Check sheet for the modelled part. Datum: model origin and axes. Units: mm. A direction names the side the tool comes from. Give positions to 0.01 mm unless a question says otherwise; leave off trailing zeros. Loops run counter-clockwise (first coordinate to the right, second up) from the corner with the lowest first, then second, coordinate; pieces in that order, holes last. Notation, with made-up numbers: (55, 28) -> (64, 28) arc R25 ccw to (64, 58) -> close; hole circle Ø8 at (40.25, 57). An arc over 180 degrees is marked (long way). Write each question's results on one line, items separated by ' | '. Start each with the question number.
Item 1: Cross-section at A-A on z = 0.5. Enter the section's corners in (x, y).
Item 2: Cross-section at B-B on y = 73. Enter the section's corners in (x, z).
Item 3: Mould release check, pull along Z, two halves, no side actions. Record for faces 3 (the face through (151.457, 44.37, 0.192)), 4 (the face through (121.87, 45.63, 12.22)), 5 (the face through (126.47, 44.37, 0.02)), 6 (the face through (-53.53, 44.37, 0.02)): pulls with the +Z half, pulls with the -Z half, needs draft (parallel to the pull), parting line crosses it, or undercut.
Item 4: Gauge pin test, flat ends, axial feed: pin 1 Ø1 at (x, y) = (84, 37.5) entering from +Z; pin 2 Ø4 at (y, z) = (52.5, -2.5) entering from -X; pin 3 Ø6 at (y, z) = (68.5, 11.5) entering from +X. Record the tip position at first contact, or that the pin passes through.
Item 5: Cross-section at D-D on z = 9.5. Enter the section's corners in (x, y).
Item 6: Cross-section at C-C on x = -36. Enter the section's corners in (y, z).
Item 7: Access from +Z, -Z, +X, -X, +Y, -Y to the whole of each face (thin tool, end or side, straight path). Record for faces 1 (the face through (48, 90, -12)), 2 (the face through (119.461, 44, -2)).
Item 8: Scan lines: line 1 along X through (y, z) = (25.5, 0.5); line 2 along X through (y, z) = (29, 8.5); line 3 along Z through (x, y) = (101, 52). Record each from-to range of solid material in increasing order.
from build123d import *

# Parameters (mm, degrees)
SKETCH1_R           = 11
BOSS_EXTRUDE1_DEPTH = 90
FILLET1_R           = 8


with BuildPart() as part:
    # Sketch1 → Boss-Extrude1 (new body)
    with BuildSketch(Plane(origin=(0, 0, 0), x_dir=(1, 0, 0), z_dir=(0, 1, 0))):
        with BuildLine():
            Line((137.460581558, -14.5), (119.460581558, -14.5))
            Line((119.460581558, -14.5), (119.460581558, 10.5))
            Line((119.460581558, 10.5), (-24.539418442, 10.5))
            Line((-24.539418442, 10.5), (-24.539418442, -14.5))
            Line((-24.539418442, -14.5), (-42.539418442, -14.5))
            ThreePointArc((-42.539418442, -14.5), (-56.539418442, -0.5), (-42.539418442, 13.5))
            Line((-42.539418442, 13.5), (137.460581558, 13.5))
            ThreePointArc((137.460581558, 13.5), (151.460581558, -0.5), (137.460581558, -14.5))
        make_face()
        with Locations((-42.539418442, -0.5)):
            Circle(SKETCH1_R, mode=Mode.SUBTRACT)
        with Locations((137.460581558, -0.5)):
            Circle(SKETCH1_R, mode=Mode.SUBTRACT)
    extrude(amount=BOSS_EXTRUDE1_DEPTH)

    # Fillet1
    fillet1_edges = [part.edges().sort_by_distance(p)[0] for p in [
        (119.460581558, 45, 14.5),
        (-24.539418442, 45, 14.5),
    ]]
    fillet(fillet1_edges, radius=FILLET1_R)


solid = part.part
Answer sheet:
1) outline: (-56.54, 0) -> (-53.54, 0) -> (-53.54, 90) -> (-56.54, 90) -> close; (-31.54, 0) -> (-24.54, 0) -> (-24.54, 90) -> (-31.54, 90) -> close; (119.46, 0) -> (126.46, 0) -> (126.46, 90) -> (119.46, 90) -> close; (148.46, 0) -> (151.46, 0) -> (151.46, 90) -> (148.46, 90) -> close
2) outline: (-42.54, -13.5) -> (137.46, -13.5) arc R14 ccw to (137.46, 14.5) -> (127.46, 14.5) arc R8 ccw to (119.46, 6.5) -> (119.46, -10.5) -> (-24.54, -10.5) -> (-24.54, 6.5) arc R8 ccw to (-32.54, 14.5) -> (-42.54, 14.5) arc R14 ccw to start; hole circle Ø22 at (-42.54, 0.5); hole circle Ø22 at (137.46, 0.5)
3) face 3: parting line crosses it | face 4: pulls with the +Z half | face 5: undercut | face 6: undercut
4) pin 1: stops at z = -10.5 | pin 2: stops at x = -56.5 | pin 3: stops at x = 148.95
5) outline: (-53.26, 0) -> (-48.86, 0) -> (-48.86, 90) -> (-53.26, 90) -> close; (-36.21, 0) -> (-25.12, 0) -> (-25.12, 90) -> (-36.21, 90) -> close; (120.04, 0) -> (131.14, 0) -> (131.14, 90) -> (120.04, 90) -> close; (143.79, 0) -> (148.18, 0) -> (148.18, 90) -> (143.79, 90) -> close
6) outline: (0, -13.5) -> (90, -13.5) -> (90, -8.35) -> (0, -8.35) -> close; (0, 9.35) -> (90, 9.35) -> (90, 14.5) -> (0, 14.5) -> close
7) face 1: +Z, -Z, +X, -X, +Y | face 2: +Z, +Y, -Y
8) line 1: x = -56.54 to -53.54, -31.54 to -24.54, 119.46 to 126.46, 148.46 to 151.46 | line 2: x = -54.03 to -50.09, -34.99 to -24.79, 119.71 to 129.91, 145.01 to 148.95 | line 3: z = -13.5 to -10.5
